CAD build for the part. Positions are in the model's coordinates, mm. A direction names the side the tool comes from. Coordinates: 2 decimals unless noted, no trailing zeros. Loops run counter-clockwise (first coordinate to the right, second up) from the corner with the lowest first, then second, coordinate; pieces in that order, holes last. Notation, with made-up numbers: (-37, 49.25) -> (-25, 49.25) arc R24 cw to (-25, 74.25) -> close; hole circle Ø5 at (20, 6.25). An arc over 180 degrees is marked (long way). Answer as CSV lines item,"result". Start each with the question number.
```python
from build123d import *

# Parameters (mm, degrees)
F0_R     = 0.75
F1_DEPTH = 8
F2_R     = 19.7132732736
F3_R     = 15.261888986


with BuildPart() as f1:
    # F0 (on Top) → F1 (new body)
    with BuildSketch(Plane.XY):
        with BuildLine():
            Line((-14.586677067, 11.8301414847), (-14.586677067, 16.0179088211))
            ThreePointArc((-14.586677067, 16.0179088211), (-14.6560408436, 3.8804388779), (-4.1329702753, 9.929238244))
            ThreePointArc((-4.1329702753, 9.929238244), (-4.2473311453, 11.189386557), (-4.586677067, 12.4083601108))
            Line((-4.586677067, 12.4083601108), (-4.586677067, 11.8301414847))
            Line((-4.586677067, 11.8301414847), (-14.586677067, 11.8301414847))
        make_face()
        with BuildLine():
            Line((-14.586677067, 32.8301414847), (-14.586677067, 28.8405676668))
            ThreePointArc((-14.586677067, 28.8405676668), (-8.7563690973, 28.3450323814), (-4.586677067, 32.4501163771))
            Line((-4.586677067, 32.4501163771), (-4.586677067, 32.8301414847))
            Line((-4.586677067, 32.8301414847), (-14.586677067, 32.8301414847))
        make_face()
        with BuildLine():
            ThreePointArc((-4.586677067, 32.4501163771), (-8.7563690973, 28.3450323814), (-14.586677067, 28.8405676668))
            Line((-14.586677067, 28.8405676668), (-14.586677067, 16.0179088211))
            ThreePointArc((-14.586677067, 16.0179088211), (-8.7563690973, 16.5134441066), (-4.586677067, 12.4083601108))
            Line((-4.586677067, 12.4083601108), (-4.586677067, 32.4501163771))
        make_face()
        with BuildLine():
            ThreePointArc((-4.586677067, 32.4501163771), (-4.2473311453, 33.6690899309), (-4.1329702753, 34.929238244))
            ThreePointArc((-4.1329702753, 34.929238244), (-14.6560408436, 40.97803761), (-14.586677067, 28.8405676668))
            Line((-14.586677067, 28.8405676668), (-14.586677067, 32.8301414847))
            Line((-14.586677067, 32.8301414847), (-4.586677067, 32.8301414847))
            Line((-4.586677067, 32.8301414847), (-4.586677067, 32.4501163771))
        make_face()
        with Locations((-11.1329702753, 34.929238244)):
            Circle(F0_R, mode=Mode.SUBTRACT)
        with BuildLine():
            ThreePointArc((-4.586677067, 12.4083601108), (-8.7563690973, 16.5134441066), (-14.586677067, 16.0179088211))
            Line((-14.586677067, 16.0179088211), (-14.586677067, 11.8301414847))
            Line((-14.586677067, 11.8301414847), (-4.586677067, 11.8301414847))
            Line((-4.586677067, 11.8301414847), (-4.586677067, 12.4083601108))
        make_face()
        with Locations((-11.1329702753, 34.929238244)):
            Circle(F0_R)
    extrude(amount=F1_DEPTH)

    # F2
    f2_edges = [f1.edges().sort_by_distance(p)[0] for p in [
        (-14.586677, 16.017909, 4),
    ]]
    fillet(f2_edges, radius=F2_R)

    # F3
    f3_edges = [f1.edges().sort_by_distance(p)[0] for p in [
        (-14.586677, 28.840568, 4),
    ]]
    fillet(f3_edges, radius=F3_R)


solid = f1.part
```
Q1. Saw through at A-A (y = 18.5). List the corners of the cut face in (x, z).
Q2. Saw through at B-B (x = -14). List the corners of the cut face in (y, z), and give its area (3 significant figures).
Q3. Two-plate mould, pull along Y, no slides. Class faces 3 (the cylindrical face through (-15.475, 17.378, 4.056)), 4 (the flat face through (-11, 23, 8)): pulls with the +Y half, pulls with the -Y half, needs draft (parallel to the pull), parting line crosses it, or undercut.
Q4. Probe probe 1 along X at (y, z) = (22.5, 6.75); probe 2 along Y at (x, z) = (-17, 7); probe 3 along X at (y, z) = (35, 7.25). List the from-to ranges inside material, lowest first. Write a range as from..to.
Q5. Which spindle directions (+Z, -Z, +X, -X, +Y, -Y) get a long thin tool onto all of the face, cutting with end or side? Do faces 1 (the flat face through (-11, 23, 0)), 2 (the flat face through (-4.587, 22, 4)). Say none if no direction does.
Q6. Pin check, flat tips, straight feed: pin 1 Ø1.5 at (y, z) = (19, 5) entering from +X; pin 2 Ø3 at (x, z) = (-16, 5.5) entering from -Y; pin 3 Ø1.5 at (y, z) = (13, 1) entering from +X. Stop position of each tip, or through.
Ans:
1,outline,"(-15.16, 0) -> (-4.59, 0) -> (-4.59, 8) -> (-15.16, 8) -> close"
2,outline,"(3.54, 0) -> (41.32, 0) -> (41.32, 8) -> (3.54, 8) -> close"
2,area,"302 mm²"
3,face 3,"undercut"
3,face 4,"needs draft"
4,probe 1,"x = -14.6..-4.59"
4,probe 2,"y = 6.11..13.78, 31.11..38.75"
4,probe 3,"x = -18.13..-4.13"
5,face 1,"-Z, +X, -X, +Y, -Y"
5,face 2,"+Z, -Z, +X"
6,pin 1,"stops at x = -4.59"
6,pin 2,"stops at y = 3.79"
6,pin 3,"stops at x = -4.53"
